```python
from build123d import *

# Parameters (mm, degrees)
F1_DEPTH = 3


with BuildPart() as f1:
    # F0 (on Front) → F1 (new body)
    with BuildSketch(Plane.XZ):
        with BuildLine():
            Line((-100, 0), (0, 0))
            Line((0, 0), (0, 50))
            Line((0, 50), (-100, 50))
            Line((-100, 50), (-100, 17.3523504695))
            Line((-100, 17.3523504695), (-95.7282808558, 18.0761301251))
            add(Edge.make_bspline(
                [(-95.7282808558, 18.0761301251), (-95.3488123547, 16.081045733), (-94.0465454532, 15.1639968553)],
                knots=[0, 0, 0, 1, 1, 1], degree=2))
            add(Edge.make_bspline(
                [(-94.0465454532, 15.1639968553), (-92.7442785517, 14.2469479777), (-90.2259875899, 14.2469479777)],
                knots=[0, 0, 0, 1, 1, 1], degree=2))
            add(Edge.make_bspline(
                [(-90.2259875899, 14.2469479777), (-84.0280020719, 14.2469479777), (-84.0280020719, 17.8231511244)],
                knots=[0, 0, 0, 1, 1, 1], degree=2))
            add(Edge.make_bspline(
                [(-84.0280020719, 17.8231511244), (-84.0280020719, 19.2605318104), (-85.1060375864, 20.0970873696)],
                knots=[0, 0, 0, 1, 1, 1], degree=2))
            add(Edge.make_bspline(
                [(-85.1060375864, 20.0970873696), (-86.1840731009, 20.9336429289), (-89.3865572693, 21.738576113)],
                knots=[0, 0, 0, 1, 1, 1], degree=2))
            add(Edge.make_bspline(
                [(-89.3865572693, 21.738576113), (-92.692532847, 22.6182530928), (-94.2822758857, 23.5726738683)],
                knots=[0, 0, 0, 1, 1, 1], degree=2))
            add(Edge.make_bspline(
                [(-94.2822758857, 23.5726738683), (-95.8720189244, 24.5270946438), (-96.7056997223, 25.9012305796)],
                knots=[0, 0, 0, 1, 1, 1], degree=2))
            add(Edge.make_bspline(
                [(-96.7056997223, 25.9012305796), (-97.5393805202, 27.2753665154), (-97.5393805202, 29.2704509076)],
                knots=[0, 0, 0, 1, 1, 1], degree=2))
            add(Edge.make_bspline(
                [(-97.5393805202, 29.2704509076), (-97.5393805202, 32.449936985), (-94.7192396143, 34.390400911)],
                knots=[0, 0, 0, 1, 1, 1], degree=2))
            add(Edge.make_bspline(
                [(-94.7192396143, 34.390400911), (-91.8990987084, 36.3308648371), (-87.2477348085, 36.3308648371)],
                knots=[0, 0, 0, 1, 1, 1], degree=2))
            add(Edge.make_bspline(
                [(-87.2477348085, 36.3308648371), (-82.9700898871, 36.3308648371), (-80.3828046523, 34.7756189349)],
                knots=[0, 0, 0, 1, 1, 1], degree=2))
            add(Edge.make_bspline(
                [(-80.3828046523, 34.7756189349), (-77.7955194175, 33.2203730326), (-77.2033185749, 30.2363707285)],
                knots=[0, 0, 0, 1, 1, 1], degree=2))
            Line((-77.2033185749, 30.2363707285), (-82.3778890444, 29.0347204751))
            add(Edge.make_bspline(
                [(-82.3778890444, 29.0347204751), (-82.7746061138, 30.6503363661), (-84.0941215835, 31.6133814257)],
                knots=[0, 0, 0, 1, 1, 1], degree=2))
            add(Edge.make_bspline(
                [(-84.0941215835, 31.6133814257), (-85.4136370532, 32.5764264853), (-87.5352109457, 32.5764264853)],
                knots=[0, 0, 0, 1, 1, 1], degree=2))
            add(Edge.make_bspline(
                [(-87.5352109457, 32.5764264853), (-89.7602762476, 32.5764264853), (-91.0366702968, 31.7398709261)],
                knots=[0, 0, 0, 1, 1, 1], degree=2))
            add(Edge.make_bspline(
                [(-91.0366702968, 31.7398709261), (-92.3130643459, 30.9033153668), (-92.3130643459, 29.4486861126)],
                knots=[0, 0, 0, 1, 1, 1], degree=2))
            add(Edge.make_bspline(
                [(-92.3130643459, 29.4486861126), (-92.3130643459, 28.6035062693), (-91.8444782423, 28.0113054266)],
                knots=[0, 0, 0, 1, 1, 1], degree=2))
            add(Edge.make_bspline(
                [(-91.8444782423, 28.0113054266), (-91.3758921387, 27.419104584), (-90.4789665906, 26.9792660941)],
                knots=[0, 0, 0, 1, 1, 1], degree=2))
            add(Edge.make_bspline(
                [(-90.4789665906, 26.9792660941), (-89.5820410426, 26.5394276042), (-86.9200120121, 25.8207372612)],
                knots=[0, 0, 0, 1, 1, 1], degree=2))
            add(Edge.make_bspline(
                [(-86.9200120121, 25.8207372612), (-84.0682487312, 25.0273031225), (-82.7027370795, 24.3373603933)],
                knots=[0, 0, 0, 1, 1, 1], degree=2))
            add(Edge.make_bspline(
                [(-82.7027370795, 24.3373603933), (-81.3372254278, 23.647417664), (-80.5179184368, 22.7849892524)],
                knots=[0, 0, 0, 1, 1, 1], degree=2))
            add(Edge.make_bspline(
                [(-80.5179184368, 22.7849892524), (-79.6986114458, 21.9225608408), (-79.26739724, 20.8071534285)],
                knots=[0, 0, 0, 1, 1, 1], degree=2))
            add(Edge.make_bspline(
                [(-79.26739724, 20.8071534285), (-78.8361830342, 19.6917460162), (-78.8361830342, 18.237116762)],
                knots=[0, 0, 0, 1, 1, 1], degree=2))
            add(Edge.make_bspline(
                [(-78.8361830342, 18.237116762), (-78.8361830342, 14.3561889098), (-81.8201853383, 12.3151083357)],
                knots=[0, 0, 0, 1, 1, 1], degree=2))
            add(Edge.make_bspline(
                [(-81.8201853383, 12.3151083357), (-84.8041876424, 10.2740277616), (-90.5882075228, 10.2740277616)],
                knots=[0, 0, 0, 1, 1, 1], degree=2))
            add(Edge.make_bspline(
                [(-90.5882075228, 10.2740277616), (-95.3833094912, 10.2740277616), (-97.8987256917, 11.9730117325)],
                knots=[0, 0, 0, 1, 1, 1], degree=2))
            add(Edge.make_bspline(
                [(-97.8987256917, 11.9730117325), (-99.2313673487, 12.8731159831), (-100, 14.2855889299)],
                knots=[0, 0, 0, 0.529789725, 0.529789725, 0.529789725], degree=2))
            Line((-100, 14.2855889299), (-100, 0))
        make_face()
        Polygon((-52.5493650489, 31.8577361423), (-60.742434959, 31.8577361423), (-64.8763418119, 10.6362476945), (-70.1774017818, 10.6362476945), (-66.0434949289, 31.8577361423), (-74.2193162708, 31.8577361423), (-73.4258821321, 35.951396336), (-51.761680433, 35.951396336), align=None, mode=Mode.SUBTRACT)
        Polygon((-30.4367005758, 10.6362476945), (-35.6802653183, 10.6362476945), (-36.6691832302, 17.1044607814), (-46.3168823945, 17.1044607814), (-49.8183417456, 10.6362476945), (-55.1021531472, 10.6362476945), (-40.9640767199, 35.951396336), (-34.7085959745, 35.951396336), align=None, mode=Mode.SUBTRACT)
        with BuildLine():
            Line((-3.7704140895, 10.6362476945), (-9.6291777655, 10.6362476945))
            Line((-9.6291777655, 10.6362476945), (-13.7573350957, 20.2322011541))
            Line((-13.7573350957, 20.2322011541), (-19.9783187046, 20.2322011541))
            Line((-19.9783187046, 20.2322011541), (-21.8296650281, 10.6362476945))
            Line((-21.8296650281, 10.6362476945), (-27.1249754753, 10.6362476945))
            Line((-27.1249754753, 10.6362476945), (-22.2033840065, 35.951396336))
            Line((-22.2033840065, 35.951396336), (-10.5088547453, 35.951396336))
            add(Edge.make_bspline(
                [(-10.5088547453, 35.951396336), (-7.6513419416, 35.951396336), (-5.6131361289, 35.0717193562)],
                knots=[0, 0, 0, 1, 1, 1], degree=2))
            add(Edge.make_bspline(
                [(-5.6131361289, 35.0717193562), (-3.5749303162, 34.1920423764), (-2.5141433699, 32.5563031557)],
                knots=[0, 0, 0, 1, 1, 1], degree=2))
            add(Edge.make_bspline(
                [(-2.5141433699, 32.5563031557), (-1.4533564237, 30.9205639351), (-1.4533564237, 28.7127472014)],
                knots=[0, 0, 0, 1, 1, 1], degree=2))
            add(Edge.make_bspline(
                [(-1.4533564237, 28.7127472014), (-1.4533564237, 25.7459934655), (-3.4024446338, 23.6790400391)],
                knots=[0, 0, 0, 1, 1, 1], degree=2))
            add(Edge.make_bspline(
                [(-3.4024446338, 23.6790400391), (-5.351532844, 21.6120866127), (-8.6920055583, 21.1118781339)],
                knots=[0, 0, 0, 1, 1, 1], degree=2))
            Line((-8.6920055583, 21.1118781339), (-3.7704140895, 10.6362476945))
        make_face(mode=Mode.SUBTRACT)
    extrude(amount=F1_DEPTH)


solid = f1.part
```
Design review of the part built by this model. Coordinates are the model's own, in mm. Give positions to 0.01 mm unless a question says otherwise; leave off trailing zeros. Order: outer loops, then holes, each group sorted by start corner. A loop starts at its lowest first (then second) coordinate and runs counter-clockwise, first axis right, second up. Notation, with made-up numbers: (56, 67.25) - (98, 67.25) arc R38 ccw to (98, 105.25) - close; hole circle Ø7 at (-37, -32.75). An arc over 180 degrees is marked (long way). Use a Markdown table: item, result. Add a question column.
(1) Add section C-C on y = -1. Give the number of separate pieces and of enclosed holes in the cut face, then the cut area to 3 significant figures.
(2) Add section B-B on x = -68.5. Give the boundary of the cut face in (y, z).
(3) Add section A-A on x = -17.5. Give the boundary of the cut face in (y, z).
(4) Mouldability with a two-part tool opening along X and no side actions: class faces 1 (the face through (-6.266, -1.479, 15.947)), 2 (the face through (-100, -1, 7)), 3 (the face through (0, -1, 25)) as +X half, -X half, draft (parallel to the pull), parting line (faces both ways), or undercut.
(5) Wall thickness on probe 1 along Z at (x, y) = (-91, -0.75); probe 2 along Z at (x, y) = (-15.5, -0.5); probe 3 along X at (y, z) = (-2.5, 28): over which ranges is each line inside the solid? List them lowest first. Write a range as [from, to].
Report:
| question | item | result |
|---|---|---|
| 1 | separate pieces | 1 |
| 1 | enclosed holes | 3 |
| 1 | area | 3,780 mm² |
| 2 | outline | (-3, 0) - (0, 0) - (0, 10.64) - (-3, 10.64) - close; (-3, 19.25) - (0, 19.25) - (0, 31.86) - (-3, 31.86) - close; (-3, 35.95) - (0, 35.95) - (0, 50) - (-3, 50) - close |
| 3 | outline | (-3, 0) - (0, 0) - (0, 20.23) - (-3, 20.23) - close; (-3, 35.95) - (0, 35.95) - (0, 50) - (-3, 50) - close |
| 4 | face 1 | undercut |
| 4 | face 2 | -X half |
| 4 | face 3 | +X half |
| 5 | probe 1 | z = [0, 10.28], [14.27, 22.2], [27.27, 31.76], [35.95, 50] |
| 5 | probe 2 | z = [0, 20.23], [35.95, 50] |
| 5 | probe 3 | x = [-100, -97.45], [-91.84, -66.79], [-61.49, -45.4], [-33.37, -23.75], [-1.48, 0] |
